Geometry: see drawing. Coordinates: mm, zero at the bounding-box minimum. A direction names the side the tool comes from. Give positions to 0.01 mm unless a question says otherwise; leave off trailing zeros. Write each loop counter-clockwise with the first axis right and the second up, starting at its lowest first coordinate (ties: lowest second). Pieces come first, ordered by that corner, then holes. Notation, with made-up numbers: M 84.25,43.25 L 110.25,43.25 A17 ccw 110.25,47.25 Z; hole C -33,49.5 d2. An arc over 180 degrees is marked long. Use a Markdown table: item, result. Add a question column.
(1) Cut plane B-B (y = 10). Output: boundary loops of the cut face in (x, z), plus the area to 3 significant figures.
(2) Draft query along Z for the marked faces 3, 4 and 5. Return one class per face: released by +Z, released by -Z, zero draft, split by the parting line, or undercut.
(3) Cut plane D-D (z = 1.05). Output: boundary loops of the cut face in (x, y) (3 decimals), plus the area to 3 significant figures.
(4) Pin query (flat end, axial travel): pin 1 Ø2.5 at (x, z) = (46, 3) entering from +Y; pin 2 Ø1.5 at (x, z) = (24, 1.5) entering from +Y; pin 3 Ø8.5 at (x, y) = (40, 10) entering from +Z; pin 4 Ø2.5 at (y, z) = (47, 2) entering from +X. Return the tip coordinate at first contact, or that it passes through.
(5) Cut plane A-A (x = 10). Output: boundary loops of the cut face in (y, z) (3 decimals), plus the area to 3 significant figures.
(6) Material intervals for L1, parallel to Y at x = 10, z = 1.85 (3 decimals); L2, parallel to Y at x = 40, z = 3.9; L3, parallel to Y at x = 36, z = 2.05, sorted ascending.
(7) Cut plane C-C (y = 24.5). Output: boundary loops of the cut face in (x, z), plus the area to 3 significant figures.
(8) Reachability of the marked faces 1 and 2 from +Z, -Z, +X, -X, +Y, -Y: full face, straight path, thin tool, end or side. Return the list, or none.
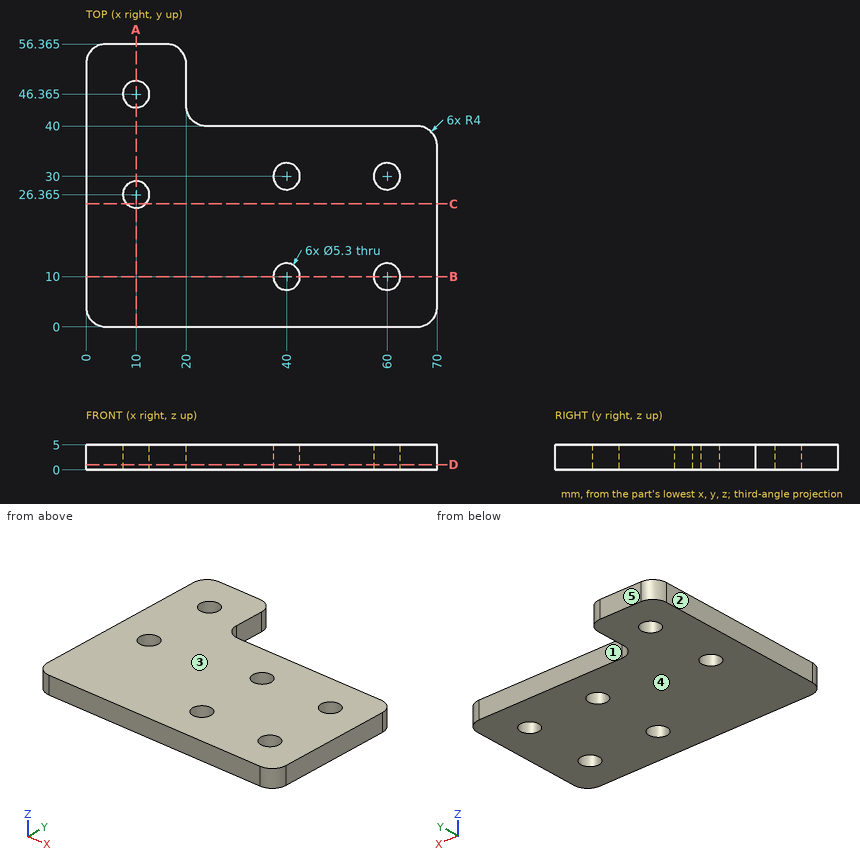
Answer list:
| question | item | result |
|---|---|---|
| 1 | outline | M 0,0 L 37.35,0 L 37.35,5 L 0,5 Z; M 42.65,0 L 57.35,0 L 57.35,5 L 42.65,5 Z; M 62.65,0 L 70,0 L 70,5 L 62.65,5 Z |
| 1 | area | 297 mm² |
| 2 | face 3 | released by +Z |
| 2 | face 4 | released by -Z |
| 2 | face 5 | zero draft |
| 3 | outline | M 0,4 A4 ccw 4,0 L 66,0 A4 ccw 70,4 L 70,36 A4 ccw 66,40 L 24,40 A4 cw 20,44 L 20,52.365 A4 ccw 16,56.365 L 4,56.365 A4 ccw 0,52.365 Z; hole C 10,26.365 d5.3; hole C 10,46.365 d5.3; hole C 40,10 d5.3; hole C 40,30 d5.3; hole C 60,10 d5.3; hole C 60,30 d5.3 |
| 3 | area | 2,980 mm² |
| 4 | pin 1 | y = 40 |
| 4 | pin 2 | y = 40.07 |
| 4 | pin 3 | z = 5 |
| 4 | pin 4 | x = 20 |
| 5 | outline | M 0,0 L 23.715,0 L 23.715,5 L 0,5 Z; M 29.015,0 L 43.715,0 L 43.715,5 L 29.015,5 Z; M 49.015,0 L 56.365,0 L 56.365,5 L 49.015,5 Z |
| 5 | area | 229 mm² |
| 6 | L1 | 0 to 23.715, 29.015 to 43.715, 49.015 to 56.365 |
| 6 | L2 | 0 to 7.35, 12.65 to 27.35, 32.65 to 40 |
| 6 | L3 | 0 to 40 |
| 7 | outline | M 0,0 L 8.12,0 L 8.12,5 L 0,5 Z; M 11.88,0 L 70,0 L 70,5 L 11.88,5 Z |
| 7 | area | 331 mm² |
| 8 | face 1 | +Z, -Z, +X, +Y |
| 8 | face 2 | +Z, -Z, -X, +Y, -Y |
